Work out the finished part from the listing and answer in its coordinate system (mm). A direction names the side the tool comes from. Coordinates: 2 decimals unless noted, no trailing zeros. Order: outer loops, then holes, each group sorted by start corner. A loop starts at its lowest first (then second) coordinate and runs counter-clockwise, first axis right, second up. Notation, with made-up numbers: (87, -19.5) -> (122, -19.5) arc R16 cw to (122, 7.5) -> close; hole circle Ø3 at (-3, 20). An arc over 180 degrees is marked (long way). Use one line per item in the form item = value.
from build123d import *

# Parameters (mm, degrees)
F1_DEPTH    = 10
F2_DEPTH    = 5
F3_T1_DEPTH = 20


# Not quite as in the source:
# - a fillet or chamfer that OpenCascade refuses, or shapes differently, is made with other operations: its cross-section is extruded or revolved along the edge and cut away or added


with BuildPart() as f1:
    # F0 (on Top) → F1 (new body)
    with BuildSketch(Plane.XY):
        with BuildLine():
            ThreePointArc((-2.8424912948, 2.0151155274), (-0.2360435678, 4.2655420814), (2.3550239983, 1.9974242942))
            Line((2.3550239983, 1.9974242942), (2.3550239983, -1.4671932394))
            ThreePointArc((2.3550239983, -1.4671932394), (-0.2360435678, -3.7353110266), (-2.8424912948, -1.4848844726))
            Line((-2.8424912948, -1.4848844726), (-3.8449760017, -1.4848844726))
            Line((-3.8449760017, -1.4848844726), (-3.8449760017, -5.2353262286))
            Line((-3.8449760017, -5.2353262286), (3.3550239983, -5.2353262286))
            Line((3.3550239983, -5.2353262286), (3.3550239983, 5.7655572834))
            Line((3.3550239983, 5.7655572834), (-3.8449760017, 5.7655572834))
            Line((-3.8449760017, 5.7655572834), (-3.8449760017, 2.0151155274))
            Line((-3.8449760017, 2.0151155274), (-2.8424912948, 2.0151155274))
        make_face()
    extrude(amount=F1_DEPTH)

    # F0 (on Top) → F2 (join)
    with BuildSketch(Plane.XY):
        with BuildLine():
            Line((2.3550239983, -1.4671932394), (2.3550239983, 1.9974242942))
            ThreePointArc((2.3550239983, 1.9974242942), (-0.2360435678, 4.2655420814), (-2.8424912948, 2.0151155274))
            Line((-2.8424912948, 2.0151155274), (-1.4057946783, 2.0151155274))
            ThreePointArc((-1.4057946783, 2.0151155274), (0.7480700142, 2.1154829532), (1.8550239983, 0.2651155274))
            ThreePointArc((1.8550239983, 0.2651155274), (0.7480700142, -1.5852518984), (-1.4057946783, -1.4848844726))
            Line((-1.4057946783, -1.4848844726), (-2.8424912948, -1.4848844726))
            ThreePointArc((-2.8424912948, -1.4848844726), (-0.2360435678, -3.7353110266), (2.3550239983, -1.4671932394))
        make_face()
    extrude(amount=F2_DEPTH)

    # F3: fillet of radius 2 on 4 edges, made by hand

    # F3_s2 → F3_t1 (cut)
    with BuildSketch(Plane.XY.offset(-5)):
        with BuildLine():
            ThreePointArc((-1.8449760017, 2.0151155274), (-3.259189564, 2.600901965), (-3.8449760017, 4.0151155274))
            Line((-3.8449760017, 4.0151155274), (-3.8449760017, 2.0151155274))
            Line((-3.8449760017, 2.0151155274), (-1.8449760017, 2.0151155274))
        make_face()
        with BuildLine():
            ThreePointArc((-1.8449760017, -1.4848844726), (-3.259189564, -2.0706709102), (-3.8449760017, -3.4848844726))
            Line((-3.8449760017, -3.4848844726), (-3.8449760017, -1.4848844726))
            Line((-3.8449760017, -1.4848844726), (-1.8449760017, -1.4848844726))
        make_face()
        with BuildLine():
            ThreePointArc((-1.8449760017, -5.2353262286), (-3.259189564, -4.6495397909), (-3.8449760017, -3.2353262286))
            Line((-3.8449760017, -3.2353262286), (-3.8449760017, -5.2353262286))
            Line((-3.8449760017, -5.2353262286), (-1.8449760017, -5.2353262286))
        make_face()
        with BuildLine():
            ThreePointArc((-1.8449760017, 5.7655572834), (-3.259189564, 5.1797708458), (-3.8449760017, 3.7655572834))
            Line((-3.8449760017, 3.7655572834), (-3.8449760017, 5.7655572834))
            Line((-3.8449760017, 5.7655572834), (-1.8449760017, 5.7655572834))
        make_face()
    extrude(amount=F3_T1_DEPTH, mode=Mode.SUBTRACT)


solid = f1.part
(1) The mould has two halves that part along Y. Classify faces 1 (the cylindrical face through (-3.199, -4.707, 4.93)), 2 (the cylindrical face through (-3.199, 5.238, 4.93)), 3 (the cylindrical face through (-3.425, -2.259, 4.93)): released by +Y, released by -Y, zero draft, split by the parting line, or undercut.
Data:
face_1 = released by -Y
face_2 = released by +Y
face_3 = undercut
(2) Each of these flat-tipped pins is pushed along its axis until it touches: P1, Ø6, axis at y = -4, z = 8.5, coming from the -X side; P2, Ø4, axis at y = -0.5, z = 8, coming from the -X side. Where does it stop, or does it pass through?
Data:
P1 = -3.84
P2 = -3.59
(3) Section B-B on z = 1.25 is taken. Write down the section's boundary in (x, y), plus the area to 3 significant figures.
Data:
outline = (-3.84, -3.36) arc R2 ccw to (-1.84, -5.24) -> (3.36, -5.24) -> (3.36, 5.77) -> (-1.84, 5.77) arc R2 ccw to (-3.84, 3.89) arc R2 ccw to (-1.84, 2.02) -> (-1.41, 2.02) arc R2.1 cw (long way) to (-1.41, -1.48) -> (-1.84, -1.48) arc R2 ccw to start
area = 55.7 mm²
(4) Section A-A on x = -1 is taken. Write down the section's boundary in (y, z).
Data:
outline = (-5.24, 0) -> (-1.69, 0) -> (-1.69, 5) -> (-3.62, 5) -> (-3.62, 10) -> (-5.24, 10) -> close; (2.22, 0) -> (5.77, 0) -> (5.77, 10) -> (4.15, 10) -> (4.15, 5) -> (2.22, 5) -> close
(5) Which of the six approach directions +Z, -Z, +X, -X, +Y, -Y give full straight-line access (tool end or side, diameter ignored) to faces 4 (the flat face through (2.355, 0, 7)), 5 (the flat face through (2, 0, 5)), 6 (the flat face through (1, 5.766, 5)), 7 (the cylindrical face through (-3.425, 2.79, 4.93))?
Data:
face_4 = +Z, -X
face_5 = +Z
face_6 = +Z, -Z, +X, -X, +Y
face_7 = +Z, -Z, -X
(6) Section D-D on x = 1.25 is taken. Write down the section's boundary in (y, z).
Data:
outline = (-5.24, 0) -> (-1.21, 0) -> (-1.21, 5) -> (-3.27, 5) -> (-3.27, 10) -> (-5.24, 10) -> close; (1.74, 0) -> (5.77, 0) -> (5.77, 10) -> (3.8, 10) -> (3.8, 5) -> (1.74, 5) -> close
(7) Straight lines are drawn through the part: line 1 along Y through (x, z) = (-0.25, 5.25); line 2 along Z through (x, y) = (2, 2); line 3 along Y through (x, z) = (-2, 8.75). For each, find the intervals that lie inside material, in ascending order.
Data:
line_1 = -5.24 to -3.74, 4.27 to 5.77
line_2 = 0 to 5
line_3 = -5.23 to -3.06, 3.59 to 5.76
(8) Section C-C on y = 3.5 is taken. Write down the section's boundary in (x, z).
Data:
outline = (-3.78, 0) -> (3.36, 0) -> (3.36, 10) -> (1.61, 10) -> (1.61, 5) -> (-2.1, 5) -> (-2.1, 10) -> (-3.78, 10) -> close
